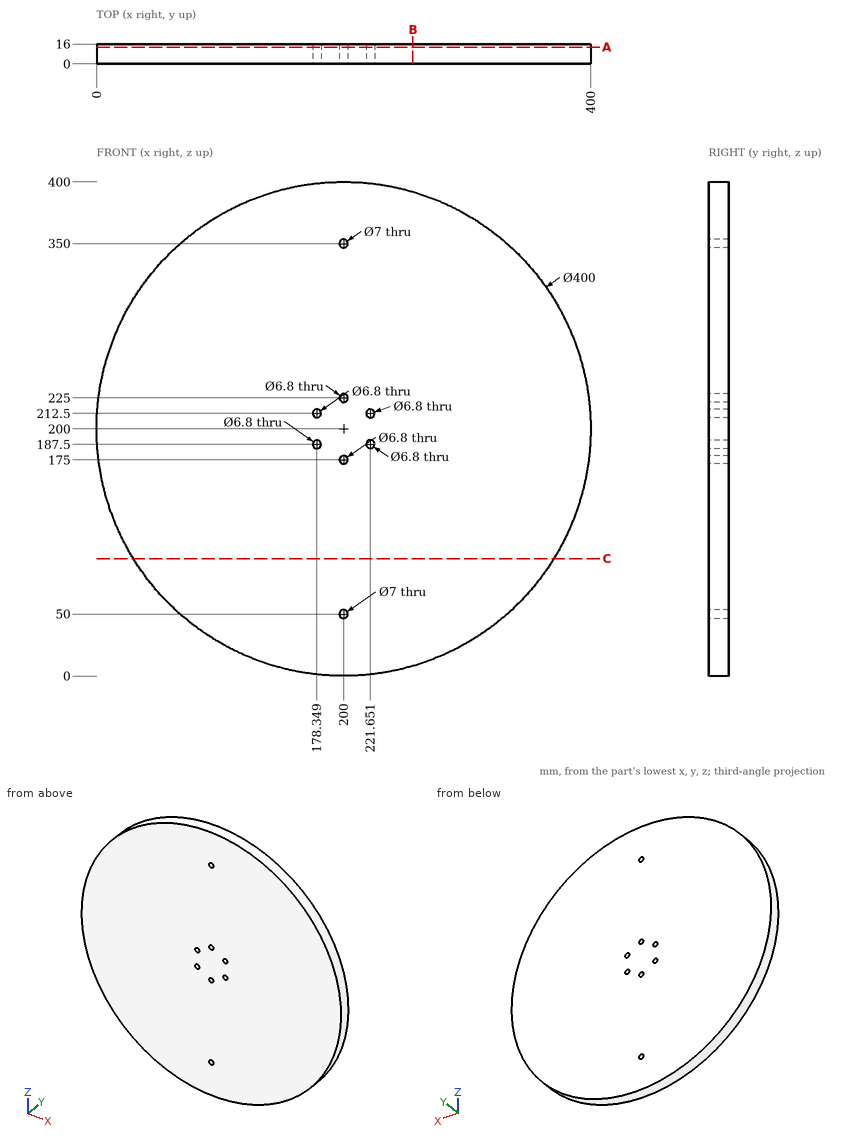
Input: dimensioned drawing with shaded views. Units: mm. Origin: part minimum x, y, z. Give positions to 0.01 mm unless a question says otherwise; leave off trailing zeros. Order: outer loops, then holes, each group sorted by start corner. A loop starts at its lowest first (then second) coordinate and runs counter-clockwise, first axis right, second up. Notation, with made-up numbers: (-16.75, 67) -> (37.25, 67) arc R15 ccw to (37.25, 72) -> close; hole circle Ø9 at (-26.75, 54.5). An arc over 180 degrees is marked (long way). Answer as a JSON object with one key per item and string values.
Q1. Section A-A (y = 13.5). State how many separate pieces and enclosed holes the cut face has, plus the area to 3 significant figures.
Entries:
{"separate pieces": "1", "enclosed holes": "8", "area": "125,000 mm^2"}
Q2. Section B-B (x = 256). Output: boundary loops of the cut face in (y, z), plus the area to 3 significant figures.
Entries:
{"outline": "(0, 8) -> (16, 8) -> (16, 392) -> (0, 392) -> close", "area": "6,140 mm^2"}
Q3. First-contact query: pin 1 (6 mm diameter, centred on x = 221.65, z = 212.5, fed in from -Y); pin 2 (11 mm diameter, centred on x = 221.65, z = 187.5, fed in from -Y); pin 3 (1.5 mm diameter, centred on y = 6, z = 104.5, fed in from +X); pin 4 (1.5 mm diameter, centred on y = 10.5, z = 288, fed in from -X) (1 decimal). Flat tips, straight axial feed; report the tip coordinate or a pass-through.
Entries:
{"pin 1": "passes through", "pin 2": "stops at y = 0", "pin 3": "stops at x = 376.13", "pin 4": "stops at x = 20"}
Q4. Material intervals for probe 1 along X at (y, z) = (11.5, 187.5); probe 2 along X at (y, z) = (6.75, 225); probe 3 along Z at (x, y) = (161, 10.5), sorted ascending.
Entries:
{"probe 1": "x = 0.39 to 174.95, 181.75 to 218.25, 225.05 to 399.61", "probe 2": "x = 1.57 to 196.6, 203.4 to 398.43", "probe 3": "z = 3.84 to 396.16"}
Q5. Section C-C (z = 95). Output: boundary loops of the cut face in (x, y).
Entries:
{"outline": "(29.78, 0) -> (370.22, 0) -> (370.22, 16) -> (29.78, 16) -> close"}
